from build123d import *

# Parameters (mm, degrees)
SKETCH040_W      = 7
SKETCH040_H      = 34
EXTRUDE049_DEPTH = 2
EXTRUDE048_DEPTH = 2


with BuildPart() as extrude049:
    # Sketch040 → Extrude049 (new body)
    with BuildSketch(Plane.XZ.offset(4.5)):
        with Locations((-37.5, 12)):
            Rectangle(SKETCH040_W, SKETCH040_H)
    extrude(amount=-EXTRUDE049_DEPTH)


with BuildPart() as bulge_overlap:
    # Sketch039 → Extrude048 (new body)
    with BuildSketch(Plane.XZ.offset(5.3)):
        Polygon((-37, 31), (-35.4, 29.4), (-35.4, -5.4), (-37, -7), (-39.9, -7), (-39.9, 31), align=None)
    extrude(amount=-EXTRUDE048_DEPTH)

    # Cut027: cut Extrude049
    add(extrude049.part, mode=Mode.SUBTRACT)


with BuildPart() as bulge_overlap_1:
    # Cut027 placement: moved
    add(bulge_overlap.part.moved(Location((40, 0, 0))))


solid = bulge_overlap_1.part
Could you check a few things on this model? Use its own coordinates, in mm. A direction names the side the tool comes from. Give positions to 0.01 mm unless a question says otherwise; leave off trailing zeros. Order: outer loops, then holes, each group sorted by start corner. A loop starts at its lowest first (then second) coordinate and runs counter-clockwise, first axis right, second up.
Item 1: I'm going to push a flat-ended pin straight in: pin 1 (1 mm diameter, centred on x = 1, z = 3.5, fed in from +Y). Where does the tip first touch, or does it pass through?
Item 2: For faces 1 (the face through (2, -4, -5)), 2 (the face through (2, -5.3, 12)), which set-ups out of +Z, -Z, +X, -X, +Y, -Y let a thin tool reach every point of the face, with its end or its side?
Item 3: If we mould it in two halves opening along Z, with no side actions, what happens to faces 3 (the face through (2, -4, 29)), 4 (the face through (2, -4, -7)), 5 (the face through (2, -3.3, -6))? For each: pulls with the +Z half, pulls with the -Z half, needs draft (parallel to the pull), parting line crosses it, or undercut.
Item 4: If we section it at C-C, the plane z = 22: Write out the boundary of the cut face in (x, y).
Item 5: If we section it at A-A, the plane x = 1.1: Write out the boundary of the cut face in (y, z).
Item 6: If we section it at D-D, the plane x = 3.4: Write out the boundary of the cut face in (y, z).
Item 7: I need wall thicknesses on line 1 (Z direction, x = 0.9, y = -4.1); line 2 (Y direction, x = 1.4, z = 12); line 3 (Z direction, x = 3.35, y = -3.85). Which ranges of each line are inside material? Lowest first, please.
Item 8: If we section it at B-B, the plane y = -4.15: Write out the boundary of the cut face in (x, z).
Values:
1. pin 1: stops at y = -4.5
2. face 1: +X, -X, +Y
2. face 2: +Z, -Z, +X, -X, -Y
3. face 3: undercut
3. face 4: pulls with the -Z half
3. face 5: needs draft
4. outline: (0.1, -5.3) - (4.6, -5.3) - (4.6, -4.5) - (0.1, -4.5) - close
5. outline: (-5.3, -7) - (-3.3, -7) - (-3.3, -5) - (-4.5, -5) - (-4.5, 29) - (-3.3, 29) - (-3.3, 31) - (-5.3, 31) - close
6. outline: (-5.3, -6.6) - (-3.3, -6.6) - (-3.3, -5) - (-4.5, -5) - (-4.5, 29) - (-3.3, 29) - (-3.3, 30.6) - (-5.3, 30.6) - close
7. line 1: z = -7 to -5, 29 to 31
7. line 2: y = -5.3 to -4.5
7. line 3: z = -6.65 to -5, 29 to 30.65
8. outline: (0.1, -7) - (3, -7) - (4.6, -5.4) - (4.6, -5) - (0.1, -5) - close; (0.1, 29) - (4.6, 29) - (4.6, 29.4) - (3, 31) - (0.1, 31) - close
